Autodesk Inventor part; units mm, degrees
ref_plane "YZ Plane" through (0, 0, 0) normal (1, 0, 0) x (0, 1, 0)
ref_plane "XZ Plane" through (0, 0, 0) normal (0, 1, 0) x (-1, 0, 0)
ref_plane "XY Plane" through (0, 0, 0) normal (0, 0, 1) x (1, 0, 0)
sketch "Sketch1" plane through (0, 0, 0) normal (0, 1, 0) x (-1, 0, 0)
  line L0 (14.75, -8) -> (9.75, -8)
  line L1 (9.75, -8) -> (9.75, 8)
  line L2 (9.75, 8) -> (14.75, 8)
  line L3 (14.75, 8) -> (14.75, -8)
  line L4 (-14.75, -8) -> (-9.75, -8)
  line L5 (-9.75, -8) -> (-9.75, 8)
  line L6 (-9.75, 8) -> (-14.75, 8)
  line L7 (-14.75, 8) -> (-14.75, -8)
  line L8 (0, -17.6647) -> (0, 17.6647)
  line L9 (27.0734, 0) -> (-27.0734, 0)
  line L10 (18.75, -12) -> (-18.75, -12)
  line L11 (-18.75, -12) -> (-18.75, 12)
  line L12 (-18.75, 12) -> (18.75, 12)
  line L13 (18.75, 12) -> (18.75, -12)
  arc A0 (5.8816, -6.8013) -> (18.75, -5.5) centre (12.25, -5.5) ccw
  arc A1 (-18.75, -5.5) -> (-5.8816, -6.8013) centre (-12.25, -5.5) ccw
  arc A2 (5.8816, -6.8013) -> (-5.8816, -6.8013) centre (0, -8.0031) ccw
  arc A3 (18.75, 5.5) -> (5.8816, 6.8013) centre (12.25, 5.5) ccw
  arc A4 (-5.8816, 6.8013) -> (-18.75, 5.5) centre (-12.25, 5.5) ccw
  arc A5 (-5.8816, 6.8013) -> (5.8816, 6.8013) centre (0, 8.0031) ccw
  point P0 (0, 0)
  point P1 (0, -2)
  point P2 (-18.75, 5.5)
  dimension "d0" = 5
  dimension "d1" = 16
  dimension "d2" = 16
  dimension "d3" = 19.5
  dimension "d4" = 37.5
  dimension "d5" = 24
  dimension "d6" = 6.5
  dimension "d7" = 4
  dimension "d8" = 2
extrude "Extrusion1" add sketch "Sketch1" against normal blind 72 contours L3 L9 L13 A0 A2 L8 L1 L0 | L3 L2 L1 L9 L8 A5 A3 L13 | L9 L5 L6 L7 L11 A4 A5 L8 | L8 A2 A1 L11 L9 L7 L4 L5
sketch "Sketch2" plane through (0, -72, 0) normal (0, -1, 0) x (1, 0, 0)
  arc A0 (-5.8816, 6.8013) -> (-18.75, 5.5) centre (-12.25, 5.5) ccw
  line L0 (-18.75, 5.5) -> (-18.75, -5.5)
  arc A1 (-18.75, -5.5) -> (-5.8816, -6.8013) centre (-12.25, -5.5) ccw
  arc A2 (5.8816, -6.8013) -> (-5.8816, -6.8013) centre (0, -8.0031) ccw
  arc A3 (5.8816, -6.8013) -> (18.75, -5.5) centre (12.25, -5.5) ccw
  line L1 (18.75, -5.5) -> (18.75, 5.5)
  arc A4 (18.75, 5.5) -> (5.8816, 6.8013) centre (12.25, 5.5) ccw
  arc A5 (-5.8816, 6.8013) -> (5.8816, 6.8013) centre (0, 8.0031) ccw
  line L2 (-14.75, -8) -> (-14.75, 8)
  line L3 (-14.75, 8) -> (-9.75, 8)
  line L4 (-9.75, 8) -> (-9.75, -8)
  line L5 (-9.75, -8) -> (-14.75, -8)
  line L6 (9.75, -8) -> (9.75, 8)
  line L7 (9.75, 8) -> (14.75, 8)
  line L8 (14.75, 8) -> (14.75, -8)
  line L9 (14.75, -8) -> (9.75, -8)
  line L10 (15.9006, 9.0344) -> (8.0535, 9.0344)
  line L11 (8.0535, 9.0344) -> (8.0535, -9.2409)
  line L12 (8.0535, -9.2409) -> (15.9006, -9.2409)
  line L13 (15.9006, -9.2409) -> (15.9006, 9.0344)
  line L14 (-8.673, 9.0344) -> (-16.1071, 9.0344)
  line L15 (-16.1071, 9.0344) -> (-16.1071, -9.2409)
  line L16 (-16.1071, -9.2409) -> (-8.673, -9.2409)
  line L17 (-8.673, -9.2409) -> (-8.673, 9.0344)
  point P0 (0, 0)
extrude "Extrusion2" add sketch "Sketch2" against normal blind 56 contours L2 L3 L4 L5 | L6 L7 L8 L9 | L13 L12 L11 L10 | L17 L16 L15 L14
sketch "Sketch3" plane through (0, -72, 0) normal (0, -1, 0) x (1, 0, 0)
  line L0 (-44.45, 0) -> (44.45, 0)
  line L1 (0, -44.3994) -> (0, 45.8962)
  arc A0 (-6.3941, -26.1683) -> (6.3941, -26.1683) centre (0, -25) ccw
  circle A1 centre (0, 25) radius 6.5
  arc A2 (-5.8816, 6.8013) -> (-18.75, 5.5) centre (-12.25, 5.5) ccw
  line L2 (-18.75, 5.5) -> (-18.75, -5.5)
  arc A3 (-18.75, -5.5) -> (-5.8816, -6.8013) centre (-12.25, -5.5) ccw
  arc A4 (5.8816, -6.8013) -> (-5.8816, -6.8013) centre (0, -8.0031) ccw
  arc A5 (5.8816, -6.8013) -> (18.75, -5.5) centre (12.25, -5.5) ccw
  line L3 (18.75, -5.5) -> (18.75, 5.5)
  arc A6 (18.75, 5.5) -> (5.8816, 6.8013) centre (12.25, 5.5) ccw
  arc A7 (-5.8816, 6.8013) -> (5.8816, 6.8013) centre (0, 8.0031) ccw
  arc A8 (26.3546, -6.4055) -> (26.3546, 6.4055) centre (25.25, 0) ccw
  arc A9 (-26.3546, 6.4055) -> (-26.3546, -6.4055) centre (-25.25, 0) ccw
  arc A10 (26.3546, -6.4055) -> (6.3941, -26.1683) centre (30.5229, -30.5769) ccw
  arc A11 (6.3941, 26.1683) -> (26.3546, 6.4055) centre (30.5229, 30.5769) ccw
  arc A12 (-6.3941, -26.1683) -> (-26.3546, -6.4055) centre (-30.5229, -30.5769) ccw
  arc A13 (-26.3546, 6.4055) -> (-6.3941, 26.1683) centre (-30.5229, 30.5769) ccw
  arc A14 (0, 31.5) -> (6.3941, 26.1683) centre (0, 25) ccw
  point P0 (0, 0)
  point P1 (6.3941, 26.1683)
  point P2 (-6.3941, 26.1683)
  dimension "d14" = 13
  dimension "d13" = 13
  dimension "d15" = 13
  dimension "d16" = 50
  dimension "d17" = 50.5
extrude "Extrusion3" add sketch "Sketch3" against normal blind 3
sketch "Sketch4" plane through (0, -69, 0) normal (0, 1, 0) x (1, 0, 0)
  arc A0 (-6.3941, -26.1683) -> (6.3941, -26.1683) centre (0, -25) ccw
  point P0 (0, 0)
hole "Hole1" at (0, -69, 25) direction (0, -1, 0) diameter 4.4 end through all
sketch "Sketch5" plane through (0, -69, 0) normal (0, 1, 0) x (1, 0, 0)
  arc A0 (6.3941, 26.1683) -> (-6.3941, 26.1683) centre (0, 25) ccw
  point P0 (0, 0)
hole "Hole2" at (0, -69, -25) direction (0, -1, 0) diameter 4.4 end through all
sketch "Sketch6" plane through (0, 0, 0) normal (0, 0, 1) x (1, 0, 0)
  line L0 (31.75, -69) -> (26.3546, -69)
  line L1 (16.0779, -69) -> (26.3546, -69)
  line L2 (18.75, 0) -> (18.75, -69)
  line L3 (31.75, -72) -> (31.75, -69)
  line L4 (0, -86.4) -> (0, 14.4)
  line L5 (29.0523, -70.5) -> (29.0523, -69)
  line L6 (29.0523, -69) -> (18.75, -58.6977)
  line L7 (29.0523, -69) -> (43.622, -69) construction
  line L8 (18.75, -58.6977) -> (17.25, -58.6977)
  line L9 (17.25, -58.6977) -> (17.25, -70.5)
  line L10 (17.25, -70.5) -> (29.0523, -70.5)
  line L11 (-29.0523, -70.5) -> (-29.0523, -69)
  line L12 (-29.0523, -69) -> (-18.75, -58.6977)
  line L13 (-18.75, -58.6977) -> (-17.25, -58.6977)
  line L14 (-17.25, -58.6977) -> (-17.25, -70.5)
  line L15 (-17.25, -70.5) -> (-29.0523, -70.5)
  point P0 (0, 0)
  dimension "d34" = 135
  dimension "d35" = 1.5
  dimension "d36" = 1.5
extrude "Extrusion4" add sketch "Sketch6" along normal mid plane 3
properties part number "pilar soporte"
Source: CAD feature listing. Evaluate the final solid. Frame: model axes, mm. A direction names the side the tool comes from. Coordinates: 2 decimals unless noted, no trailing zeros. Loops run counter-clockwise (first coordinate to the right, second up) from the corner with the lowest first, then second, coordinate; pieces in that order, holes last. Notation, with made-up numbers: M 12.5,-33 L 31.5,-33 A13 ccw 31.5,-29 Z; hole C 65.5,61 d2. An arc over 180 degrees is marked long. Put each result on its own line as item: value. Start each with the question number.
1) Cut plane B-B on y = -18. Return the cut outline in (x, z).
2) Contact query for flat-ended pins moving along their axis: pin 1 Ø5.5 at (x, y) = (-13, -6) entering from +Z; pin 2 Ø1.5 at (x, y) = (-13.5, -50.5) entering from -Z; pin 3 Ø2 at (x, y) = (-14.5, -22.5) entering from -Z; pin 4 Ø3.5 at (x, z) = (0, 25) entering from +Y. Output: stop coordinate, or through.
3) Cut plane A-A on x = 0. Return the cut outline in (y, z).
4) Ray query, L1, parallel to Z at x = 0, y = -70.3; L2, parallel to Y at x = -7, z = -10.5; L3, parallel to X at y = -70.9, z = -25. Return the intervals inside material, ascending. Write a range as from..to.
5) Pull-direction query (X, two-part tool) for faces 5 (the face through (-13.04, -34.02, 11.95)), 6 (the face through (18.75, -34, 0)), 7 (the face through (-18.75, -34, 0)), 8 (the face through (-22, -66, 1.5)); classes: pulls with the +X half, pulls with the -X half, needs draft (parallel to the pull), parting line crosses it, or undercut.
6) Cut plane D-D on x = -8. Return the cut outline in (y, z).
7) Cut plane C-C on z = -25. Return the cut outline in (x, y), then the cut area to 3 significant figures.
8) Reachability of faces 1 (the face through (6, -69, -13)), 2 (the face through (22, -66, 1.5)), 3 (the face through (-22, -66, -1.5)), 4 (the face through (0, -34, -2)) from +Z, -Z, +X, -X, +Y, -Y: full face, straight path, thin tool, end or side. Return the list, or none.
The answers:
1. outline: M -18.75,-5.5 A6.5 ccw -5.88,-6.8 A6 cw 5.88,-6.8 A6.5 ccw 18.75,-5.5 L 18.75,5.5 A6.5 ccw 5.88,6.8 A6 cw -5.88,6.8 A6.5 ccw -18.75,5.5 Z
2. pin 1: stops at z = 12
2. pin 2: stops at z = -11.98
2. pin 3: stops at z = -11.88
2. pin 4: passes through
3. outline: M -72,-31.5 L -69,-31.5 L -69,-27.2 L -72,-27.2 Z; M -72,-22.8 L -69,-22.8 L -69,-2 L 0,-2 L 0,2 L -69,2 L -69,22.8 L -72,22.8 Z; M -72,27.2 L -69,27.2 L -69,31.5 L -72,31.5 Z
4. L1: z = -31.5..-27.2, -22.8..22.8, 27.2..31.5
4. L2: y = -72..-69
4. L3: x = -6.64..-2.2, 2.2..6.64
5. face 5: undercut
5. face 6: pulls with the +X half
5. face 7: pulls with the -X half
5. face 8: needs draft
6. outline: M -72,-20.86 L -69,-20.86 L -69,-10.42 L 0,-10.42 L 0,10.42 L -69,10.42 L -69,20.86 L -72,20.86 Z
7. outline: M -6.64,-72 L -2.2,-72 L -2.2,-69 L -6.64,-69 Z; M 2.2,-72 L 6.64,-72 L 6.64,-69 L 2.2,-69 Z
7. area: 26.6 mm²
8. face 1: +Y
8. face 2: +Z, +X, +Y
8. face 3: -Z, -X, +Y
8. face 4: -Z, +Y
